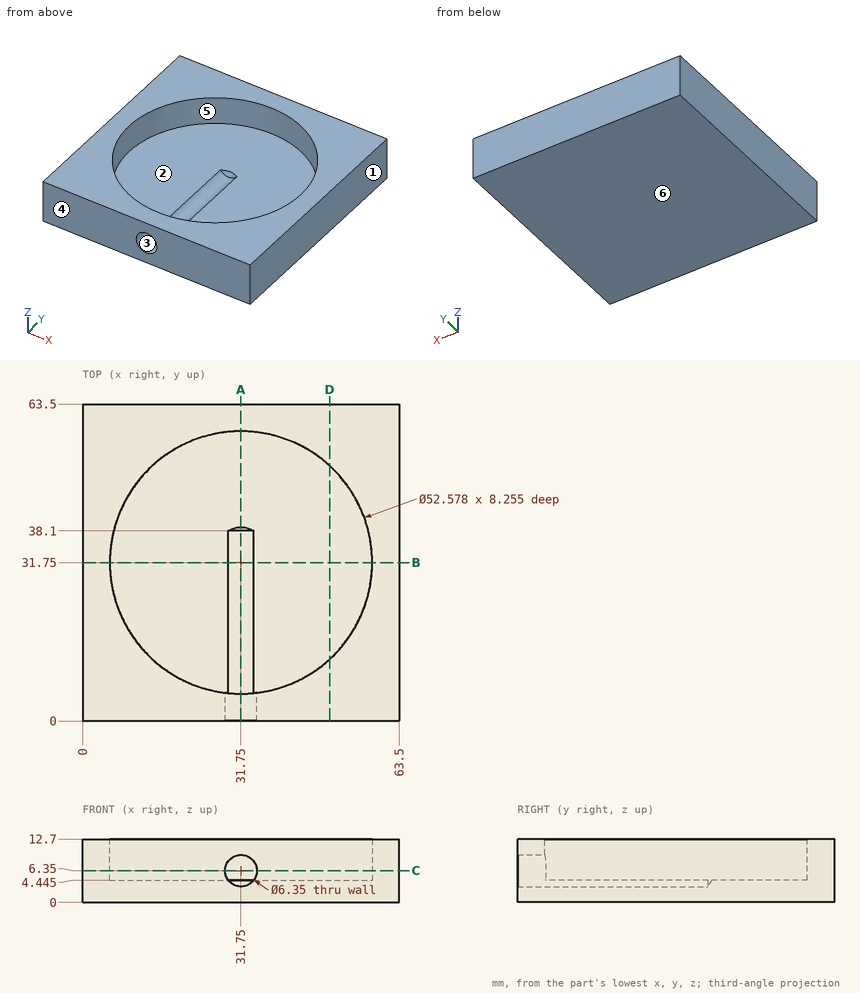
Design review of the part shown in the three views and the two pictorial views. Dimensions are in mm from the part's minimum x, y and z. A direction names the side the tool comes from. Give positions to 0.01 mm unless a question says otherwise; leave off trailing zeros. Write each loop counter-clockwise with the first axis right and the second up, starting at its lowest first coordinate (ties: lowest second). Pieces come first, ordered by that corner, then holes. Notation, with made-up numbers: M 50.25,54 L 79.25,54 A21 cw 79.25,85 Z; hole C 59.5,67 d9. An arc over 180 degrees is marked long. Return JSON: item names as keys, results as strings. Group by question number.
Item 1: Tool access review of the marked faces 1, 2 and 3: name each direction out of +Z, -Z, +X, -X, +Y, -Y from which nothing blocks a thin tool from reaching the whole face with its end or side.
Item 2: Take a section at A-A (x = 31.75). Give the boundary of the cut face in (y, z) (3 decimals), plus the area to 3 significant figures.
Item 3: Take a section at B-B (y = 31.75). Give the boundary of the cut face in (x, z) (3 decimals), plus the area to 3 significant figures.
Item 4: The part is to be moulded in two halves that separate along Y. For the marked faces 4, 5 and 6, say which applies: pulls with the +Y half, pulls with the -Y half, needs draft (parallel to the pull), parting line crosses it, or undercut.
Item 5: Wall thickness on line 1 along Y through (x, z) = (31, 10.25); line 2 along Z through (x, y) = (31.75, 20.5) (3 decimals); line 3 along Z through (x, y) = (25, 22) (3 decimals): over which ranges is each line inside the solid? List them lowest first.
Item 6: Take a section at C-C (z = 6.35). Give the boundary of the cut face in (x, y) (3 decimals).
Item 7: Take a section at D-D (x = 49.5). Give the boundary of the cut face in (y, z) (3 decimals), plus the area to 3 significant figures.
Item 8: Clearance check with flat-ended pins moving along their axes: pin 1 Ø4 at (x, z) = (31.75, 6.35) entering from -Y; pin 2 Ø5 at (x, y) = (33, 36) entering from +Z (3 decimals). State where each tip first meets the part, or that it passes through.
Return value:
{
 "1": {"face 1": "+Z, -Z, +X, +Y, -Y", "face 2": "+Z", "face 3": "-Y"},
 "2": {"outline": "M 0,0 L 63.5,0 L 63.5,12.7 L 58.039,12.7 L 58.039,4.445 L 38.863,4.445 L 38.1,3.175 L 0,3.175 Z; M 0,9.525 L 5.461,9.525 L 5.461,12.7 L 0,12.7 Z", "area": "296 mm2"},
 "3": {"outline": "M 0,0 L 63.5,0 L 63.5,12.7 L 58.039,12.7 L 58.039,4.445 L 34.29,4.445 A3.175 cw 29.21,4.445 L 5.461,4.445 L 5.461,12.7 L 0,12.7 Z", "area": "368 mm2"},
 "4": {"face 4": "pulls with the -Y half", "face 5": "undercut", "face 6": "needs draft"},
 "5": {"line 1": "y = 0 to 5.47, 58.03 to 63.5", "line 2": "z = 0 to 3.175", "line 3": "z = 0 to 4.445"},
 "6": {"outline": "M 0,0 L 28.575,0 L 28.575,5.653 A26.289 cw long 34.925,5.653 L 34.925,0 L 63.5,0 L 63.5,63.5 L 0,63.5 Z"},
 "7": {"outline": "M 0,0 L 63.5,0 L 63.5,12.7 L 51.142,12.7 L 51.142,4.445 L 12.358,4.445 L 12.358,12.7 L 0,12.7 Z", "area": "486 mm2"},
 "8": {"pin 1": "stops at y = 38.81", "pin 2": "stops at z = 4.445"}
}
